The model under review builds one solid part; all positions refer to its coordinate system, in mm. Face numbers are marked on the shaded views. A direction names the side the tool comes from. Coordinates: 2 decimals unless noted, no trailing zeros. Order: outer loops, then holes, each group sorted by start corner. A loop starts at its lowest first (then second) coordinate and runs counter-clockwise, first axis right, second up. Notation, with made-up numbers: M 78,72.5 L 85,72.5 A20 cw 85,92.5 Z; hole C -39.75,54 d5. An arc over 180 degrees is marked long. One line per item, written item: value.
Autodesk Inventor part; units mm, degrees
ref_plane "YZ Plane" through (0, 0, 0) normal (1, 0, 0) x (0, 1, 0)
ref_plane "XZ Plane" through (0, 0, 0) normal (0, 1, 0) x (-1, 0, 0)
ref_plane "XY Plane" through (0, 0, 0) normal (0, 0, 1) x (1, 0, 0)
sketch "Sketch1" plane through (0, 0, 0) normal (1, 0, 0) x (0, 1, 0)
  line L0 (-46, 60) -> (46, 60)
  line L1 (46, 60) -> (46, -60)
  line L2 (46, -60) -> (-46, -60)
  line L3 (-46, -60) -> (-46, 60)
  line L4 (-46, 60) -> (46, -60) construction
  line L5 (46, 60) -> (-46, -60) construction
  point P0 (0, 0)
  dimension "d0" = 92
  dimension "d1" = 120
extrude "Extrusion1" add sketch "Sketch1" along normal blind 10
sketch "Sketch3" plane through (10, 0, 0) normal (1, 0, 0) x (0, 0, -1)
  circle A0 centre (0, 18) radius 32
  line L0 (-60, -46) -> (60, -46)
  point P0 (0, 0)
  point P1 (0, -46)
  dimension "d16" = 64
  dimension "d17" = 64
extrude "Extrusion3" cut sketch "Sketch3" against normal through all
fillet "Fillet1" radius 8 2 edges at (5, 46, 15.4919) (5, 46, -15.4919)
sketch "Sketch6" plane through (0, -46, -60) normal (0, -1, 0) x (1, 0, 0)
  circle A0 centre (5, 114) radius 2
  line L0 (10, 120) -> (10, 0) construction
  circle A1 centre (5, 102) radius 2
  circle A2 centre (5, 90) radius 2
  circle A3 centre (5, 78) radius 2
  circle A4 centre (5, 66) radius 2
  circle A5 centre (5, 54) radius 2
  circle A6 centre (5, 42) radius 2
  circle A7 centre (5, 30) radius 2
  circle A8 centre (5, 18) radius 2
  circle A9 centre (5, 6) radius 2
  line L1 (5, 66) -> (5, 54) construction
  line L2 (0, 120) -> (0, 0)
  line L3 (0, 120) -> (10, 120)
  point P0 (0, 60)
  point P1 (5, 60)
  point P2 (0, 60)
  point P3 (5, 120)
  dimension "d66" = 4
  dimension "d69" = 12
extrude "Extrusion6" cut sketch "Sketch6" against normal blind 8
sketch "Sketch7" plane through (10, 0, 0) normal (1, 0, 0) x (0, 0, -1)
  circle A0 centre (-52, 38) radius 2.06
  line L0 (-34.641, 46) -> (-60, 46) construction
  line L1 (-60, 46) -> (-60, -46) construction
  line L2 (60, 46) -> (34.641, 46) construction
  line L3 (60, -46) -> (60, 46) construction
  line L4 (-60, -46) -> (60, -46)
  line L5 (0, 0) -> (0, -46) construction
  circle A1 centre (52, 38) radius 2.06
  circle A2 centre (-52, 6) radius 2.06
  circle A3 centre (-52, -26) radius 2.06
  circle A4 centre (52, 6) radius 2.06
  circle A5 centre (52, -26) radius 2.06
  dimension "d76" = 4.12
  dimension "d78" = 8
  dimension "d84" = 84
  dimension "d87" = 32
extrude "Extrusion7" cut sketch "Sketch7" against normal through all
properties part number "FirstStageMotorSupportPlate" material "Aluminum 6061"
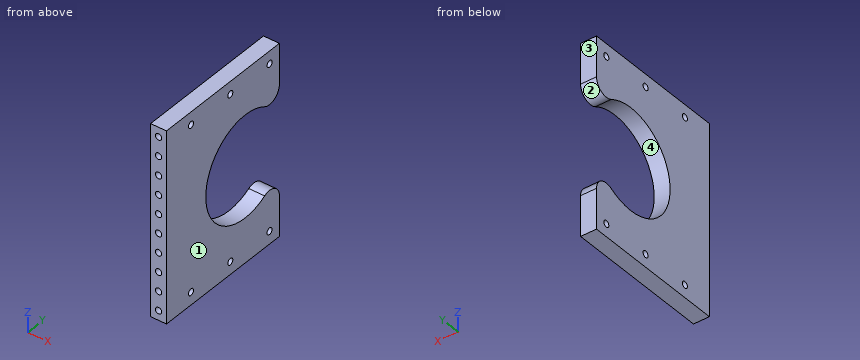
(1) Insertion check: pin 1 Ø6.5 at (y, z) = (38, 52) entering from +X; pin 2 Ø2.5 at (x, z) = (5, 54) entering from -Y; pin 3 Ø4 at (x, z) = (4, 22) entering from +Y; pin 4 Ø3.5 at (y, z) = (6, 52) entering from +X. Each pin has a flat end and moves straight along its axis. Give the tip position at first contact, or say it passes through.
Geometry results:
pin 1: stops at x = 10
pin 2: stops at y = -38
pin 3: stops at y = -3.17
pin 4: passes through
(2) Mouldability with a two-part tool opening along Z and no side actions: class the marked faces 3 and 4 as +Z half, -Z half, draft (parallel to the pull), parting line (faces both ways), or undercut.
Geometry results:
face 3: draft
face 4: undercut
(3) We need section A-A, the plane y = -26. State the section outline as (x, z) points.
Geometry results:
outline: M 0,-60 L 10,-60 L 10,-54.06 L 0,-54.06 Z; M 0,-49.94 L 10,-49.94 L 10,49.94 L 0,49.94 Z; M 0,54.06 L 10,54.06 L 10,60 L 0,60 Z
(4) For L1, parallel to Z at x = 6.5, y = 18; L2, parallel to Z at x = 7, y = 39.5; L3, parallel to Y at x = 1, z = -52.5, list the stretches that pass through material, from the lowest coordinate up.
Geometry results:
L1: z = -60 to -32, 32 to 60
L2: z = -60 to -53.41, -50.59 to -26.78, 26.78 to 50.59, 53.41 to 60
L3: y = -46 to -28, -24 to 4, 8 to 36, 40 to 46
(5) We need section B-B, the plane z = 30. State the section outline as (x, y) points, plus the area to 3 significant figures.
Geometry results:
outline: M 0,-46 L 3,-46 L 3,-38 L 7,-38 L 7,-46 L 10,-46 L 10,6.86 L 0,6.86 Z; M 0,29.14 L 10,29.14 L 10,44.52 L 0,44.52 Z
area: 650 mm2
(6) We need section D-D, the plane x = 1.5. State the section outline as (y, z) points, plus the area to 3 significant figures.
Geometry results:
outline: M -46,-60 L 46,-60 L 46,-34.64 A8 ccw 34,-27.71 A32 cw long 34,27.71 A8 ccw 46,34.64 L 46,60 L -46,60 Z; hole C -26,-52 d4.12; hole C -26,52 d4.12; hole C 6,-52 d4.12; hole C 6,52 d4.12; hole C 38,-52 d4.12; hole C 38,52 d4.12
area: 7,700 mm2
(7) We need section C-C, the plane y = 18. State the section outline as (x, z) points, plus the area to 3 significant figures.
Geometry results:
outline: M 0,-60 L 10,-60 L 10,-32 L 0,-32 Z; M 0,32 L 10,32 L 10,60 L 0,60 Z
area: 560 mm2
(8) Tool access review of the marked faces 1 and 2: name each direction out of +Z, -Z, +X, -X, +Y, -Y from which nothing blocks a thin tool from reaching the whole face with its end or side.
Geometry results:
face 1: +Z, -Z, +X, +Y, -Y
face 2: +X, -X
